Could you check a few things on this model? Use its own coordinates, in mm. A direction names the side the tool comes from. Coordinates: 2 decimals unless noted, no trailing zeros. Write each loop counter-clockwise with the first axis right and the second up, starting at its lowest first coordinate (ties: lowest second). Pieces come first, ordered by that corner, then holes. Notation, with made-up numbers: M 12,-4.75 L 34,-4.75 A18 cw 34,30.25 Z; hole C 18,-9 d5. An arc over 180 degrees is marked long. Write item = value, one per line.
Autodesk Inventor part; units mm, degrees
ref_plane "YZ Plane" through (0, 0, 0) normal (1, 0, 0) x (0, 1, 0)
ref_plane "XZ Plane" through (0, 0, 0) normal (0, 1, 0) x (-1, 0, 0)
ref_plane "XY Plane" through (0, 0, 0) normal (0, 0, 1) x (1, 0, 0)
sketch "Sketch1" plane through (0, 0, 0) normal (0, 1, 0) x (-1, 0, 0)
  line L0 (52.3087, -21.6726) -> (-32.6913, -21.6726)
  line L1 (-32.6913, -21.6726) -> (-32.6913, 48.3274)
  line L2 (-32.6913, 48.3274) -> (52.3087, 48.3274)
  line L3 (52.3087, 48.3274) -> (52.3087, -21.6726)
  dimension "d4" = 70
  dimension "d5" = 85
extrude "Extrusion1" add sketch "Sketch1" along normal blind 30
sketch "Sketch2" plane through (0, 30, 0) normal (0, 1, 0) x (1, 0, 0)
  line L0 (32.6913, 21.6726) -> (-52.3087, 21.6726)
  line L1 (-52.3087, 21.6726) -> (-52.3087, -48.3274)
  line L2 (-52.3087, -48.3274) -> (32.6913, -48.3274)
  line L3 (32.6913, -48.3274) -> (32.6913, 21.6726)
  line L4 (-52.3087, 21.6726) -> (32.6913, 21.6726)
  line L5 (32.6913, 21.6726) -> (32.6913, -43.3274)
  line L6 (32.6913, -43.3274) -> (-52.3087, -43.3274)
  line L7 (-52.3087, -43.3274) -> (-52.3087, 21.6726)
  point P0 (0, 0)
  dimension "d8" = 0
  dimension "d9" = 0
  dimension "d10" = 5
extrude "Extrusion2" cut sketch "Sketch2" against normal blind 25 contours L3 L6 L1 L0
sketch "Sketch3" plane through (0, 5, 0) normal (0, 1, 0) x (1, 0, 0)
  line L0 (-52.3087, -43.3274) -> (-52.3087, 21.6726)
  line L1 (32.6913, -43.3274) -> (-52.3087, -43.3274)
  line L2 (32.6913, 21.6726) -> (32.6913, -43.3274)
  line L3 (-34.9087, 4.0726) -> (15.2913, 4.0726)
  line L4 (15.2913, 4.0726) -> (15.2913, -21.4274)
  line L5 (15.2913, -21.4274) -> (-34.9087, -21.4274)
  line L6 (-34.9087, -21.4274) -> (-34.9087, 4.0726)
  line L7 (-52.3087, 21.6726) -> (32.6913, 21.6726)
  line L8 (-52.3087, -48.3274) -> (-52.3087, 21.6726)
  line L9 (-9.8087, -43.3274) -> (-9.8087, 21.6726) construction
  circle A0 centre (-39.3087, -25.6774) radius 1.625
  circle A1 centre (-39.3087, 8.3226) radius 1.625
  circle A2 centre (19.6913, 8.3226) radius 1.625
  circle A3 centre (19.6913, -25.6774) radius 1.625
  line L10 (-34.9087, -8.6774) -> (15.2913, -8.6774) construction
  point P0 (0, 0)
  dimension "d14" = 17.4
  dimension "d15" = 17.4
  dimension "d17" = 21.9
  dimension "d106" = 25.5
  dimension "d107" = 3.25
  dimension "d110" = 34
  dimension "d111" = 59
extrude "Extrusion3" cut sketch "Sketch3" against normal blind 1.5 contours L3 L4 L5 L6 | A0 | A1 | A2 | A3
sketch "Sketch4" plane through (0, 3.5, 0) normal (0, 1, 0) x (1, 0, 0)
  line L0 (-34.9087, 4.0726) -> (15.2913, 4.0726)
  line L1 (-34.9087, -21.4274) -> (-34.9087, 4.0726)
  line L2 (15.2913, -21.4274) -> (-34.9087, -21.4274)
  line L3 (15.2913, 4.0726) -> (15.2913, -21.4274)
  line L4 (-32.9087, 2.0726) -> (11.2913, 2.0726)
  line L5 (11.2913, 2.0726) -> (11.2913, -19.4274)
  line L6 (11.2913, -19.4274) -> (-32.9087, -19.4274)
  line L7 (-32.9087, -19.4274) -> (-32.9087, 2.0726)
  point P0 (0, 0)
  dimension "d20" = 2
  dimension "d21" = 2
  dimension "d22" = 2
  dimension "d23" = 4
extrude "Extrusion4" cut sketch "Sketch4" against normal blind 1 contours L4 L5 L6 L7
sketch "Sketch10" plane through (32.6913, 5, 43.3274) normal (0, 0, -1) x (-1, 0, 0)
  line L0 (85, 25) -> (85, 0)
  line L1 (0, 25) -> (85, 25)
  circle A0 centre (18, 9.75) radius 3.5
  circle A1 centre (67, 9.75) radius 3.5
  point P0 (32.6913, -5)
  dimension "d53" = 15.25
  dimension "d55" = 15.25
  dimension "d58" = 7
  dimension "d59" = 7
  dimension "d70" = 49
  dimension "d71" = 18
extrude "Extrusion9" cut sketch "Sketch10" against normal blind 5
sketch "Sketch16" plane through (15.2913, 5, -4.0726) normal (-1, 0, 0) x (0, 0, 1)
  line L0 (0, 0) -> (25.5, 0)
  line L1 (0, 0) -> (0, -1.5)
  line L2 (0, -1.5) -> (25.5, -1.5)
  line L3 (25.5, 0) -> (25.5, -1.5)
  point P0 (4.0726, -5)
sketch "Sketch17" plane through (0, 2.5, 0) normal (0, 1, 0) x (1, 0, 0)
  line L0 (-32.9087, 2.0726) -> (11.2913, 2.0726)
  line L1 (-32.9087, -19.4274) -> (-32.9087, 2.0726)
  line L2 (11.2913, -19.4274) -> (-32.9087, -19.4274)
  line L3 (11.2913, 2.0726) -> (11.2913, -19.4274)
  line L4 (-32.9087, 2.0726) -> (11.2913, 2.0726)
  line L5 (11.2913, 2.0726) -> (11.2913, -19.4274)
  line L6 (11.2913, -19.4274) -> (-32.9087, -19.4274)
  line L7 (-32.9087, -19.4274) -> (-32.9087, 2.0726)
  point P0 (0, 0)
  dimension "d93" = 0
  dimension "d94" = 0
  dimension "d95" = 0
  dimension "d96" = 0
extrude "Extrusion14" cut sketch "Sketch17" along normal through all both and the other way through all
sketch "Sketch20" plane through (32.6913, 0, 48.3274) normal (1, 0, 0) x (0, 0, -1)
  line L0 (19.65, 3.5) -> (25.65, 3.5)
  line L1 (25.65, 3.5) -> (25.65, 1)
  line L2 (25.65, 1) -> (19.65, 1)
  line L3 (19.65, 1) -> (19.65, 3.5)
  line L4 (21.025, 3.5) -> (24.275, 3.5) construction
  line L5 (55.025, 3.5) -> (58.275, 3.5) construction
  line L6 (53.65, 3.5) -> (59.65, 3.5)
  line L7 (59.65, 3.5) -> (59.65, 1)
  line L8 (59.65, 1) -> (53.65, 1)
  line L9 (53.65, 1) -> (53.65, 3.5)
  point P0 (48.3274, 0)
  dimension "d113" = 2.5
  dimension "d125" = 6
  dimension "d139" = 1.375
  dimension "d140" = 1.375
extrude "Extrusion16" cut sketch "Sketch20" against normal blind 16
sketch "Sketch21" plane through (-52.3087, 0, -21.6726) normal (-1, 0, 0) x (0, 0, 1)
  line L0 (17.6, 3.5) -> (43.1, 3.5)
  line L1 (10.35, 1.5) -> (16.35, 1.5)
  line L2 (16.35, 1.5) -> (16.35, 3.5)
  line L3 (16.35, 3.5) -> (10.35, 3.5)
  line L4 (10.35, 3.5) -> (10.35, 1.5)
  line L5 (44.35, 1) -> (50.35, 1)
  line L6 (50.35, 1) -> (50.35, 3.5)
  line L7 (50.35, 3.5) -> (44.35, 3.5)
  line L8 (44.35, 3.5) -> (44.35, 1)
  line L9 (10.35, 3.5) -> (10.35, 1.5)
  line L10 (10.35, 1.5) -> (16.35, 1.5)
  line L11 (16.35, 1.5) -> (16.35, 3.5)
  line L12 (50.35, 1) -> (50.35, 3.5)
  line L13 (44.35, 1) -> (50.35, 1)
  line L14 (44.35, 3.5) -> (44.35, 1)
  point P0 (21.6726, 0)
extrude "Extrusion17" cut sketch "Sketch21" against normal blind 16
sketch "Sketch22" plane through (0, 5, 0) normal (0, 1, 0) x (1, 0, 0)
  circle A0 centre (-39.3087, -25.6774) radius 1.625
  circle A1 centre (19.6913, 8.3226) radius 1.625
  circle A2 centre (-39.3087, 8.3226) radius 1.625
  circle A3 centre (19.6913, -25.6774) radius 1.625
  circle A4 centre (19.6913, 8.3226) radius 1.625
  circle A5 centre (19.6913, -25.6774) radius 1.625
  circle A6 centre (-39.3087, 8.3226) radius 1.625
  circle A7 centre (-39.3087, -25.6774) radius 1.625
  point P0 (0, 0)
extrude "Extrusion18" cut sketch "Sketch22" against normal through all
properties part number "SampleBase"
Item 1: For faces 1 (the face through (-10, 5, 25)), 2 (the face through (25, 2, 28.677)), 3 (the face through (-44, 2, -5.323)), which set-ups out of +Z, -Z, +X, -X, +Y, -Y let a thin tool reach every point of the face, with its end or its side?
Numbers:
face_1 = -Z, +X, -X, +Y
face_2 = +X
face_3 = -X
Item 2: Imagine slicing it at B-B (x = -45). Write out the boundary of the cut face in (y, z), and give its area (3 significant figures).
Numbers:
outline = M 0,-21.67 L 5,-21.67 L 5,43.33 L 30,43.33 L 30,48.33 L 0,48.33 Z; hole M 1,22.68 L 3.5,22.68 L 3.5,28.68 L 1,28.68 Z; hole M 1.5,-11.32 L 3.5,-11.32 L 3.5,-5.32 L 1.5,-5.32 Z
area = 448 mm²
Item 3: If we mould it in two halves opening along Z, with no side actions, what happens to faces 4 (the face through (-44, 3, -11.323)), 5 (the face through (-9, 15, 48.327)), 6 (the face through (-9, 0, 22))? For each: pulls with the +Z half, pulls with the -Z half, needs draft (parallel to the pull), parting line crosses it, or undercut.
Numbers:
face_4 = undercut
face_5 = pulls with the +Z half
face_6 = needs draft
Item 4: Imagine slicing it at A-A (y = 14.75). Write out the boundary of the cut face in (x, z).
Numbers:
outline = M -52.31,43.33 L -37.81,43.33 L -37.81,48.33 L -52.31,48.33 Z; M -30.81,43.33 L 11.19,43.33 L 11.19,48.33 L -30.81,48.33 Z; M 18.19,43.33 L 32.69,43.33 L 32.69,48.33 L 18.19,48.33 Z
Item 5: Imagine slicing it at D-D (z = 33). Write out the boundary of the cut face in (x, y), and give its area (3 significant figures).
Numbers:
outline = M -52.31,0 L 32.69,0 L 32.69,5 L -52.31,5 Z
area = 425 mm²
Item 6: I'm going to push flat-ended pins straight in: P1, Ø1.5, axis at x = -22, z = 22.5, coming from the +Y side; P2, Ø2, axis at x = -8.5, y = 14, coming from the -Z side; P3, Ø1.9, axis at x = -39.31, z = -8.32, coming from the -Y side; P4, Ø1.2, axis at y = 2.5, z = -7.5, coming from the +X side. Where does each tip first touch, or does it pass through?
Numbers:
P1 = 5
P2 = 43.33
P3 = through
P4 = 16.69
Item 7: Imagine slicing it at C-C (x = 1.5). Write out the boundary of the cut face in (y, z), and give its area (4 significant figures).
Numbers:
outline = M 0,-21.67 L 5,-21.67 L 5,-4.07 L 3.5,-4.07 L 3.5,-2.07 L 0,-2.07 Z; M 0,19.43 L 3.5,19.43 L 3.5,21.43 L 5,21.43 L 5,43.33 L 30,43.33 L 30,48.33 L 0,48.33 Z
area = 361.5 mm²
Item 8: If I drill on line 1 along Y through (x, z) = (26.5, 26.5); line 2 along Z through (x, y) = (12, 25); line 3 along Y through (x, z) = (10, 30.5), over which ranges is the centre line in solid material (lowest first)?
Numbers:
line_1 = 0 to 1, 3.5 to 5
line_2 = 43.33 to 48.33
line_3 = 0 to 5
